Input: part model. Units: mm. Frame: model coordinates. Face numbers are marked on the shaded views. Coordinates: 2 decimals unless noted, no trailing zeros. Answer as a JSON object with one key per item and string values.
from build123d import *

# Parameters (mm, degrees)
SKETCH1_W           = 137
SKETCH1_H           = 47
BOSS_EXTRUDE1_DEPTH = 25
FILLET1_R           = 4
SKETCH2_W           = 8
SKETCH2_H           = 8
CUT_EXTRUDE1_DEPTH  = 4.5
FILLET2_R           = 5
SKETCH3_R           = 2
CUT_EXTRUDE2_DEPTH  = 10


with BuildPart() as part:
    # Sketch1 → Boss-Extrude1 (new body)
    with BuildSketch(Plane(origin=(0, 0, 0), x_dir=(1, 0, 0), z_dir=(0, 1, 0))):
        Rectangle(SKETCH1_W, SKETCH1_H)
    extrude(amount=BOSS_EXTRUDE1_DEPTH)

    # Fillet1
    fillet1_edges = [part.edges().sort_by_distance(p)[0] for p in [
        (-68.5, 12.5, 23.5),
        (68.5, 12.5, 23.5),
        (68.5, 12.5, -23.5),
        (-68.5, 12.5, -23.5),
    ]]
    fillet(fillet1_edges, radius=FILLET1_R)

    # Sketch2 → Cut-Extrude1 (cut)
    with BuildSketch(Plane(origin=(0, 25, 0), x_dir=(1, 0, 0), z_dir=(0, 1, 0))):
        with Locations((64.5, 19.5)):
            Rectangle(SKETCH2_W, SKETCH2_H)
        with Locations((64.5, -19.5)):
            Rectangle(SKETCH2_W, SKETCH2_H)
    extrude(amount=-CUT_EXTRUDE1_DEPTH, mode=Mode.SUBTRACT)

    # Fillet2
    fillet2_edges = [part.edges().sort_by_distance(p)[0] for p in [
        (60.5, 22.75, -15.5),
        (60.5, 22.75, 15.5),
    ]]
    fillet(fillet2_edges, radius=FILLET2_R)

    # Sketch3 → Cut-Extrude2 (cut)
    with BuildSketch(Plane(origin=(0, 20.5, 0), x_dir=(1, 0, 0), z_dir=(0, 1, 0))):
        with Locations(Location((64.5, 19.5, 0), (0, 0, 270))):
            Circle(SKETCH3_R)
        with Locations(Location((64.5, -19.5, 0), (0, 0, 90))):
            Circle(SKETCH3_R)
    extrude(amount=-CUT_EXTRUDE2_DEPTH, mode=Mode.SUBTRACT)


solid = part.part
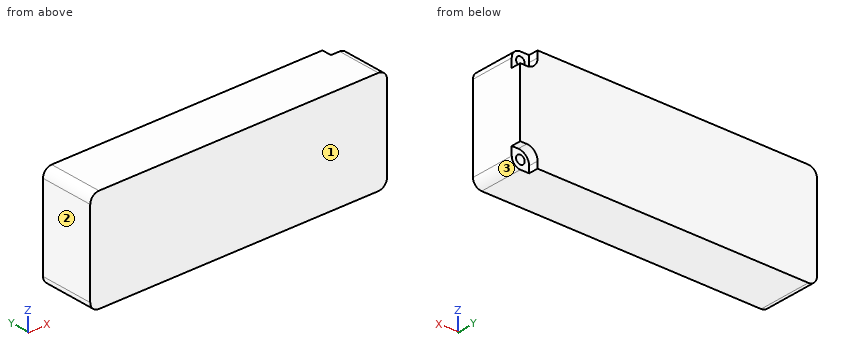
1. Line query: line 1 along X through (y, z) = (12.75, -19.5); line 2 along Y through (x, z) = (62, -19.5). Output: solid intervals per line, ascending.
Reply:
{"line 1": "x = -68.5 to 62.5, 66.5 to 68.5", "line 2": "y = 0 to 20.5"}
2. Mould query, pull axis X, two halves, no side actions, for the marked faces 1, 2 and 3. Classes: pulls with the +X half, pulls with the -X half, needs draft (parallel to the pull), parting line crosses it, or undercut.
Reply:
{"face 1": "needs draft", "face 2": "pulls with the -X half", "face 3": "pulls with the +X half"}
3. Pin query (flat end, axial travel): P1, Ø2, axis at x = 64, z = 19, coming from the +Y side; P2, Ø1.5, axis at x = 67, y = 22.5, coming from the -Z side; P3, Ø0.9, axis at y = 22.5, z = -22, coming from the +X side. Return the tip coordinate at first contact, or that it passes through.
Reply:
{"P1": "stops at y = 10.5", "P2": "stops at z = -15.5", "P3": "stops at x = 60.5"}
